Part model, mm, in its own coordinate system. Give positions to 0.01 mm unless a question says otherwise; leave off trailing zeros. Write each loop counter-clockwise with the first axis right and the second up, starting at its lowest first coordinate (ties: lowest second). Pieces come first, ordered by that corner, then holes.
Autodesk Inventor part; units mm, degrees
ref_plane "YZ Plane" through (0, 0, 0) normal (1, 0, 0) x (0, 1, 0)
ref_plane "XZ Plane" through (0, 0, 0) normal (0, 1, 0) x (-1, 0, 0)
ref_plane "XY Plane" through (0, 0, 0) normal (0, 0, 1) x (1, 0, 0)
sketch "Sketch1" plane through (0, 0, 0) normal (0, 0, 1) x (1, 0, 0)
  line L0 (35, -35) -> (-35, -35)
  line L1 (-35, -35) -> (-35, 35)
  line L2 (-35, 35) -> (35, 35)
  line L3 (35, 35) -> (35, -35)
  line L4 (35, 35) -> (-35, -35) construction
  point P0 (0, 0)
  point P1 (0, 0)
  dimension "d1" = 70
  dimension "d2" = 70
extrude "Plate1" add sketch "Sketch1" along normal blind 3
sketch "Sketch2" plane through (0, 0, 0) normal (0, 0, 1) x (1, 0, 0)
  line L0 (28, -28) -> (-28, -28) construction
  line L1 (-28, -28) -> (-28, 28) construction
  line L2 (-28, 28) -> (28, 28) construction
  line L3 (28, 28) -> (28, -28) construction
  line L4 (28, -28) -> (-28, 28) construction
  line L5 (-28, -28) -> (28, 28) construction
  circle A0 centre (-28, -28) radius 4
  circle A1 centre (28, -28) radius 4
  circle A2 centre (28, 28) radius 4
  circle A3 centre (-28, 28) radius 4
  line L6 (28, 0) -> (-28, 0) construction
  line L7 (-20, 20) -> (20, 20) construction
  line L8 (20, 20) -> (20, -20) construction
  line L9 (20, -20) -> (-20, -20) construction
  line L10 (-20, -20) -> (-20, 20) construction
  line L11 (-20, 20) -> (20, -20) construction
  line L12 (20, 20) -> (-20, -20) construction
  line L13 (-35, -35) -> (-35, 35)
  line L14 (35, -35) -> (-35, -35)
  line L15 (35, 35) -> (35, -35)
  line L16 (-35, 35) -> (35, 35)
  point P0 (0, 0)
  point P1 (75, 0)
  point P2 (0, 0)
  dimension "d7" = 8
  dimension "d33" = 40
  dimension "d35" = 7
extrude "Extrusion1" cut sketch "Sketch2" along normal through all contours A0 | A1 | A2 | A3
fillet "Corner Round1" radius 6 4 edges at (-35, 35, 1.5) (35, 35, 1.5) (35, -35, 1.5) (-35, -35, 1.5)
equation "\"d1\" = d2"
equation "\"d0\" = Thickness"
equation "\"BendRadius\" = Thickness"
equation "\"BendReliefWidth\" = Thickness"
equation "\"BendReliefDepth\" = 0.5 * Thickness"
equation "\"CornerReliefSize\" = 4 * Thickness"
equation "\"MinimumRemnant\" = 2 * Thickness"
equation "\"TransitionRadius\" = BendRadius"
equation "\"JacobiRadiusSize\" = BendRadius"
equation "\"GapSize\" = Thickness"
properties part number "GNH 018  Plate pulse pillar" material "Stainless Steel"
1) Drill centre lines: L1, parallel to X at y = -28, z = 2.1; L2, parallel to Y at x = -27, z = 2. Where is each one in solid material? Low to high.
Check result:
L1: x = -35 to -32, -24 to 24, 32 to 35
L2: y = -35 to -31.87, -24.13 to 24.13, 31.87 to 35
2) Mould opens along X. For faces 1 (the cylindrical face through (-33.289, -33.196, 1.521)), 2 (the cylindrical face through (-28.521, -31.966, 1.479)), 3 (the flat face through (0, 35, 1)) say: +X half, -X half, draft (parallel to the pull), parting line (faces both ways), or undercut.
Check result:
face 1: -X half
face 2: undercut
face 3: draft
3) Saw through at C-C (z = 1.4). Write the cut outline in (x, y), and give its area (3 significant figures).
Check result:
outline: (-35, -29) arc R6 ccw to (-29, -35) - (29, -35) arc R6 ccw to (35, -29) - (35, 29) arc R6 ccw to (29, 35) - (-29, 35) arc R6 ccw to (-35, 29) - close; hole circle Ø8 at (-28, -28); hole circle Ø8 at (-28, 28); hole circle Ø8 at (28, -28); hole circle Ø8 at (28, 28)
area: 4,670 mm2
4) Saw through at A-A (y = 28). Write the cut outline in (x, z).
Check result:
outline: (-35, 0) - (-32, 0) - (-32, 3) - (-35, 3) - close; (-24, 0) - (24, 0) - (24, 3) - (-24, 3) - close; (32, 0) - (35, 0) - (35, 3) - (32, 3) - close
5) Flat gauge pin, fed straight in: P1, Ø5, axis at x = 28, y = 28, coming from the -Z side. Where does the tip first touch, or does it go through?
Check result:
P1: passes through
